from build123d import *

# Parameters (mm, degrees)
CROQUIS1_R              = 12.5
SALIENTE_EXTRUIR1_DEPTH = 1.5
CROQUIS2_R              = 0.75
CROQUIS4_R              = 10
SALIENTE_EXTRUIR2_DEPTH = 14
CROQUIS3_R              = 7.5
CORTAR_EXTRUIR1_DEPTH   = 25.525496937


with BuildPart() as part:
    # Croquis1 → Saliente-Extruir1 (new, symmetric)
    with BuildSketch(Plane(origin=(0, 0, 0), x_dir=(1, 0, 0), z_dir=(0, 1, 0))):
        with Locations(Location((0, 0, 0), (0, 0, 270))):
            Circle(CROQUIS1_R)
    extrude(amount=SALIENTE_EXTRUIR1_DEPTH, both=True)

    # Croquis2 → Cortar-Revolución1 (revolve, cut)
    with BuildSketch(Plane(origin=(0, 0, 0), x_dir=(0, 0, -1), z_dir=(1, 0, 0)), mode=Mode.PRIVATE) as cortar_revoluci_n1_sk:
        with Locations((12.5, 0)):
            Circle(CROQUIS2_R)
    revolve(cortar_revoluci_n1_sk.sketch.rotate(Axis((0, 1.5, 0), (0, -1, 0)), 180), axis=Axis((0, 1.5, 0), (0, -1, 0)), mode=Mode.SUBTRACT)

    # Croquis4 → Saliente-Extruir2 (add)
    with BuildSketch(Plane.XZ.offset(1.5)):
        with Locations(Location((0, 0, 0), (0, 0, 90))):
            Circle(CROQUIS4_R)
    extrude(amount=SALIENTE_EXTRUIR2_DEPTH)

    # Croquis3 → Cortar-Extruir1 (cut, through all)
    with BuildSketch(Plane(origin=(0, 1.5, 0), x_dir=(1, 0, 0), z_dir=(0, 1, 0))):
        with Locations(Location((0, 0, 0), (0, 0, 270))):
            Circle(CROQUIS3_R)
    extrude(amount=-CORTAR_EXTRUIR1_DEPTH, mode=Mode.SUBTRACT)


solid = part.part
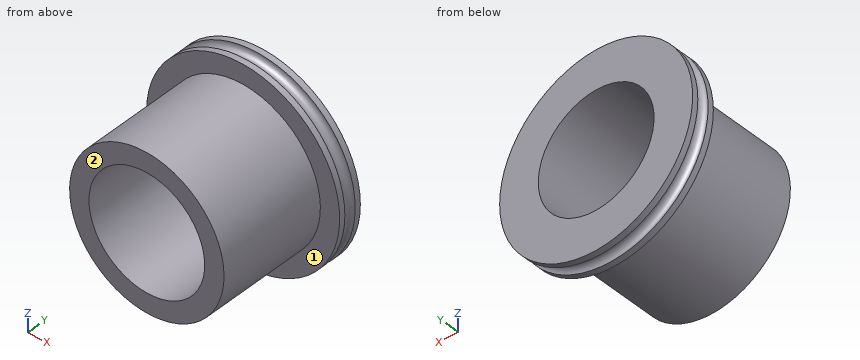
Can you work these out from the model? Positions are in its coordinate system, mm. Face numbers are marked on the shaded views. A direction names the side the tool comes from. Round coordinates to 2 decimals unless told otherwise and drop trailing zeros. Write each loop counter-clockwise with the first axis right and the second up, starting at its lowest first coordinate (ties: lowest second). Pieces come first, ordered by that corner, then holes. Notation, with made-up numbers: M 1,11.25 L 14,11.25 A18 cw 14,23.25 Z; hole C 77,57 d7. An arc over 180 degrees is marked long. Use a Markdown table: item, result.
Item 1: I want a section at A-A (x = 0). List the corners of the cut face in (y, z) for me, and give its area (3 significant figures).
Found:
| item | result |
|---|---|
| outline | M -15.5,-10 L -1.5,-10 L -1.5,-12.5 L -0.75,-12.5 A0.75 cw 0.75,-12.5 L 1.5,-12.5 L 1.5,-7.5 L -15.5,-7.5 Z; M -15.5,7.5 L 1.5,7.5 L 1.5,12.5 L 0.75,12.5 A0.75 cw -0.75,12.5 L -1.5,12.5 L -1.5,10 L -15.5,10 Z |
| area | 98.2 mm2 |
Item 2: Which directions (+Z, -Z, +X, -X, +Y, -Y) give clear straight access to the entire face, cutting with the end or side of a thin tool? Please do the marked faces 1 and 2.
Found:
| item | result |
|---|---|
| face 1 | -Y |
| face 2 | +Z, -Z, +X, -X, -Y |
Item 3: For pin 1 Ø1 at (x, y) = (-4.5, -3) entering from +Z; pin 2 Ø10 at (x, z) = (-7.5, -7.5) entering from -Y; pin 3 Ø4 at (x, y) = (-4, -5.5) entering from -Z; pin 4 Ø4 at (x, y) = (1, -11.5) entering from +Z, each with a flat end and sliding along its axis, tell me the tip position at first contact or that it passes through.
Found:
| item | result |
|---|---|
| pin 1 | stops at z = 9.17 |
| pin 2 | stops at y = -15.5 |
| pin 3 | stops at z = -9.8 |
| pin 4 | stops at z = 10 |
Item 4: If I drill on line 1 along X through (y, z) = (-10.25, 0); line 2 along Y through (x, z) = (-3.25, 10); line 3 along X through (y, z) = (-5.5, -2.25), over which ranges is the centre line in solid material (lowest first)? Write a range as [from, to].
Found:
| item | result |
|---|---|
| line 1 | x = [-10, -7.5], [7.5, 10] |
| line 2 | y = [-1.5, 1.5] |
| line 3 | x = [-9.74, -7.15], [7.15, 9.74] |
Item 5: I want a section at B-B (z = 0). List the corners of the cut face in (x, y) for me, and give its area (3 significant figures).
Found:
| item | result |
|---|---|
| outline | M -12.5,-1.5 L -10,-1.5 L -10,-15.5 L -7.5,-15.5 L -7.5,1.5 L -12.5,1.5 L -12.5,0.75 A0.75 cw -12.5,-0.75 Z; M 7.5,-15.5 L 10,-15.5 L 10,-1.5 L 12.5,-1.5 L 12.5,-0.75 A0.75 cw 12.5,0.75 L 12.5,1.5 L 7.5,1.5 Z |
| area | 98.2 mm2 |
Item 6: I want a section at C-C (y = 0). List the corners of the cut face in (x, z) for me.
Found:
| item | result |
|---|---|
| outline | C 0,0 d23.5; hole C 0,0 d15 |
Item 7: I want a section at D-D (y = -4). List the corners of the cut face in (x, z) for me, and give its area (3 significant figures).
Found:
| item | result |
|---|---|
| outline | C 0,0 d20; hole C 0,0 d15 |
| area | 137 mm2 |
